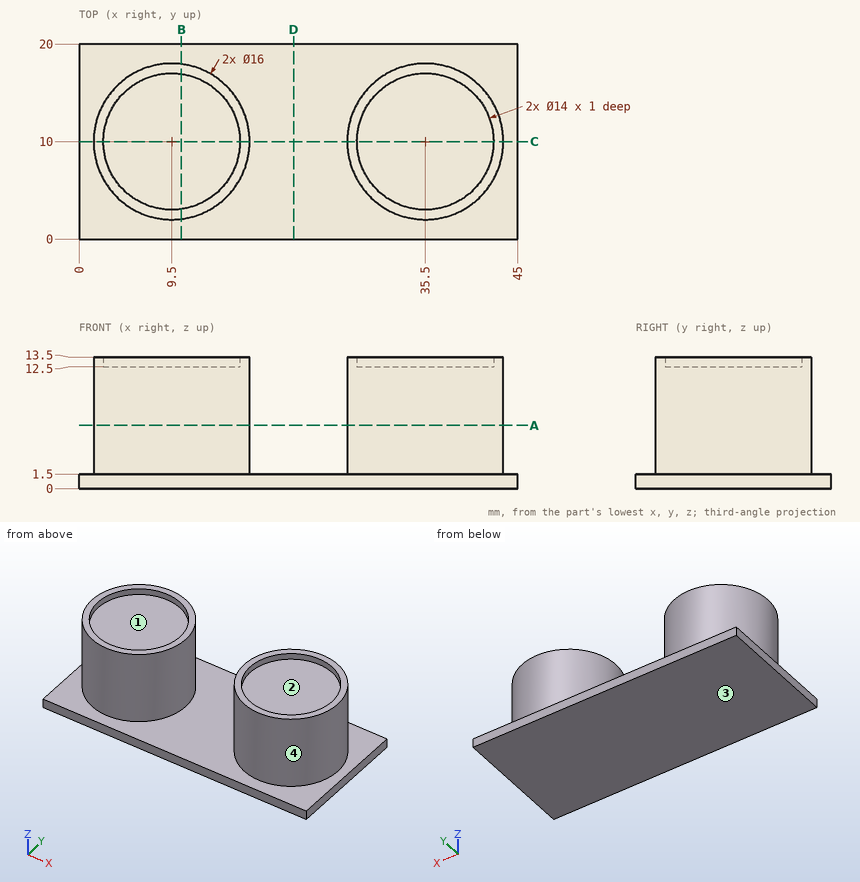
Study the drawing (mm; zero at the part's minimum x, y, z) and answer. Give positions to 0.01 mm unless a question says otherwise; leave off trailing zeros. Write each loop counter-clockwise with the first axis right and the second up, starting at its lowest first coordinate (ties: lowest second). Pieces come first, ordered by that corner, then holes. Notation, with made-up numbers: (46.25, -35) - (53.25, -35) arc R30 ccw to (53.25, -13) - close; hole circle Ø9 at (1.25, -13). An arc over 180 degrees is marked (long way). Use a Markdown table: item, result.
1. For a pull along Y with two mould halves and no side action, classify the marked faces 1, 2, 3 and 4 as released by +Y, released by -Y, zero draft, split by the parting line, or undercut.
Values follow:
| item | result |
|---|---|
| face 1 | undercut |
| face 2 | undercut |
| face 3 | zero draft |
| face 4 | split by the parting line |
2. Section D-D on x = 22 is taken. Write down the section's boundary in (y, z).
Values follow:
| item | result |
|---|---|
| outline | (0, 0) - (20, 0) - (20, 1.5) - (0, 1.5) - close |
3. Section C-C on y = 10 is taken. Write down the section's boundary in (x, z).
Values follow:
| item | result |
|---|---|
| outline | (0, 0) - (45, 0) - (45, 1.5) - (43.5, 1.5) - (43.5, 13.5) - (42.5, 13.5) - (42.5, 12.5) - (28.5, 12.5) - (28.5, 13.5) - (27.5, 13.5) - (27.5, 1.5) - (17.5, 1.5) - (17.5, 13.5) - (16.5, 13.5) - (16.5, 12.5) - (2.5, 12.5) - (2.5, 13.5) - (1.5, 13.5) - (1.5, 1.5) - (0, 1.5) - close |
4. Section B-B on x = 10.5 is taken. Write down the section's boundary in (y, z), plus the area to 3 significant figures.
Values follow:
| item | result |
|---|---|
| outline | (0, 0) - (20, 0) - (20, 1.5) - (17.94, 1.5) - (17.94, 13.5) - (16.93, 13.5) - (16.93, 12.5) - (3.07, 12.5) - (3.07, 13.5) - (2.06, 13.5) - (2.06, 1.5) - (0, 1.5) - close |
| area | 207 mm² |
5. Section A-A on z = 6.5 is taken. Write down the section's boundary in (x, y), plus the area to 3 significant figures.
Values follow:
| item | result |
|---|---|
| outline | circle Ø16 at (9.5, 10); circle Ø16 at (35.5, 10) |
| area | 402 mm² |
6. Each of these flat-tipped pins is pushed along its axis until it touches: P1, Ø4, axis at x = 34.5, y = 13, coming from the +Z side; P2, Ø2, axis at x = 30.5, z = 8, coming from the -Y side; P3, Ø1, axis at y = 14, z = 2.5, coming from the +X side; P4, Ø1, axis at x = 12, y = 16.5, coming from the +Z side. Where does it stop, or does it pass through?
Values follow:
| item | result |
|---|---|
| P1 | stops at z = 12.5 |
| P2 | stops at y = 3.07 |
| P3 | stops at x = 42.69 |
| P4 | stops at z = 13.5 |
7. Find the intervals of material crossed by probe 1 along Y at (x, z) = (9.5, 13.1); probe 2 along X at (y, z) = (15.75, 13); probe 3 along Z at (x, y) = (39, 5.5), in increasing order. Write a range as from..to.
Values follow:
| item | result |
|---|---|
| probe 1 | y = 2..3, 17..18 |
| probe 2 | x = 3.94..5.51, 13.49..15.06, 29.94..31.51, 39.49..41.06 |
| probe 3 | z = 0..12.5 |
